For this review, use the dimensioned drawing (mm, ordinates from the lowest corner) and the shaded views. A direction names the side the tool comes from. Give positions to 0.01 mm unless a question says otherwise; leave off trailing zeros. Order: outer loops, then holes, each group sorted by start corner. A loop starts at its lowest first (then second) coordinate and runs counter-clockwise, first axis right, second up. Notation, with made-up numbers: (81, 17) - (113, 17) arc R27 cw to (113, 36) - close; hole circle Ø4 at (-5, 81). An arc over 180 degrees is marked (long way). Use a Markdown table: item, result. Add a question column.
1) Clearance check with flat-ended pins moving along their axes: P1, Ø2, axis at x = 4, y = 44, coming from the +Z side; P2, Ø5, axis at x = 9, y = 37, coming from the +Z side; P3, Ø1, axis at y = 2, z = 5.5, coming from the -X side. State where each tip first meets the part, or that it passes through.
2) We need section B-B on y = 12. Write out the cut boundary in (x, z), then the cut area to 3 significant figures.
3) Wall thickness on L1, parallel to Y at x = 8.5, z = 6.5; L2, parallel to Y at x = 11.5, z = 4.75; L3, parallel to Z at x = 8.25, y = 39.5 (1 decimal): over which ranges is each line inside the solid? List them lowest first.
4) Machinability: for the marked faces 1, 2 and 3, which of the approach directions +Z, -Z, +X, -X, +Y, -Y give a long, thin tool a straight path to every point of the face, cutting with its end or side? Answer none if there is none.
5) We need section A-A on y = 44.5. Write out the cut boundary in (x, z).
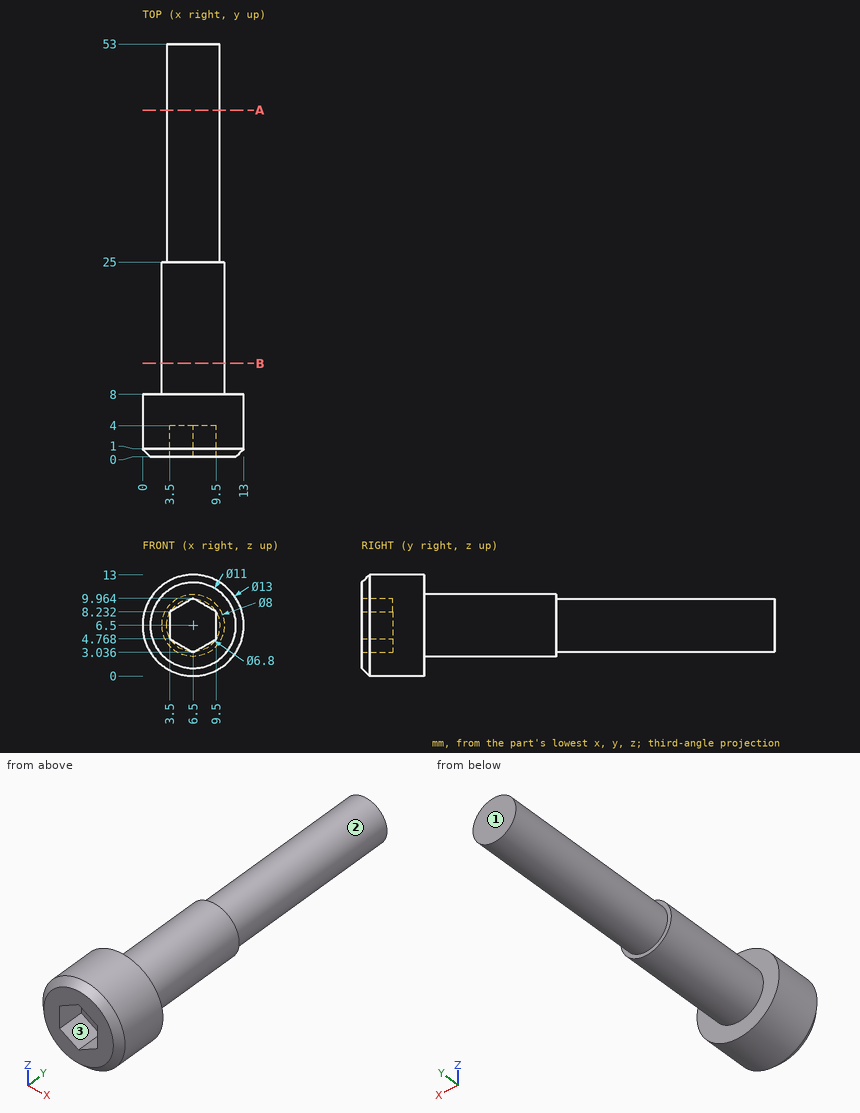
Checked values:
| question | item | result |
|---|---|---|
| 1 | P1 | z = 9.55 |
| 1 | P2 | z = 9.9 |
| 1 | P3 | x = 0.02 |
| 2 | outline | circle Ø8 at (6.5, 6.5) |
| 2 | area | 50.3 mm² |
| 3 | L1 | 4 to 53 |
| 3 | L2 | 0 to 8 |
| 3 | L3 | 3.6 to 9.4 |
| 4 | face 1 | +Z, -Z, +X, -X, +Y |
| 4 | face 2 | +Y |
| 4 | face 3 | -Y |
| 5 | outline | circle Ø6.8 at (6.5, 6.5) |
